Verification items for the finished model (mm, model axes). Face numbers are marked on the shaded views. A direction names the side the tool comes from. Round coordinates to 2 decimals unless told otherwise and drop trailing zeros. Loops run counter-clockwise (first coordinate to the right, second up) from the corner with the lowest first, then second, coordinate; pieces in that order, holes last. Notation, with made-up numbers: M -18.5,31.5 L -6.5,31.5 A29 ccw -6.5,67.5 Z; hole C 86,-24.5 d1. An arc over 180 degrees is marked long. Answer as CSV lines item,"result".
```python
from build123d import *

# Parameters (mm, degrees)
T_LE_DE_BASE_PLI_E1_DEPTH             = 20.5
ESQUISSE8_W                           = 24
ESQUISSE8_H                           = 2
BOSS_EXTRU_1_DEPTH                    = 8.5
T_LE_PLI_E_SUR_AR_TE1_STRIP_W         = 10
T_LE_PLI_E_SUR_AR_TE1_STRIP_H         = 2
T_LE_PLI_E_SUR_AR_TE1_STRIP_CUT_DEPTH = 8.5
T_LE_PLI_E_SUR_AR_TE1_DEPTH           = 8.5
ESQUISSE12_W                          = 1.5
ESQUISSE12_H                          = 12
ENL_V_MAT_EXTRU_1_DEPTH               = 8.5
DIAM_TRE_DU_PER_AGE_4_0_4_1_D         = 4
DIAM_TRE_DU_PER_AGE_4_0_4_2_D         = 4
CONG_1_R                              = 4
DIAM_TRE_DU_PER_AGE_8_0_8_2_D         = 8
DIAM_TRE_DU_PER_AGE_2_5_2_5_3_D       = 2.5
R_P_TITION_CIRCULAIRE2_COUNT          = 4


# Sheet-metal steps are written as plain solids
with BuildPart() as part:
    # Esquisse1 → Tôle de base pliée1 (new body)
    with BuildSketch(Plane(origin=(0, 0, 0), x_dir=(0, 0, -1), z_dir=(1, 0, 0))):
        with BuildLine():
            Line((0, 27), (0, 3))
            ThreePointArc((0, 3), (-0.878679656, 0.878679656), (-3, 0))
            Line((-3, 0), (-37.5, 0))
            Line((-37.5, 0), (-37.5, 2))
            Line((-37.5, 2), (-3, 2))
            ThreePointArc((-3, 2), (-2.292893219, 2.292893219), (-2, 3))
            Line((-2, 3), (-2, 27))
            Line((-2, 27), (0, 27))
        make_face()
    extrude(amount=T_LE_DE_BASE_PLI_E1_DEPTH)

    # Esquisse8 → Boss.-Extru.1 (add)
    with BuildSketch(Plane(origin=(20.5, 0, 0), x_dir=(0, 0, -1), z_dir=(1, 0, 0))):
        with Locations((-19, 1)):
            Rectangle(ESQUISSE8_W, ESQUISSE8_H)
    extrude(amount=BOSS_EXTRU_1_DEPTH)

    # Tôle pliée sur arête1 strip (across the edge) → Tôle pliée sur arête1 strip cut (cut)
    with BuildSketch(Plane(origin=(20.5, 2, 31), x_dir=(0, 0, -1), z_dir=(1, 0, 0))):
        with Locations((-4, -1)):
            Rectangle(T_LE_PLI_E_SUR_AR_TE1_STRIP_W, T_LE_PLI_E_SUR_AR_TE1_STRIP_H)
    extrude(amount=T_LE_PLI_E_SUR_AR_TE1_STRIP_CUT_DEPTH, mode=Mode.SUBTRACT)

    # Tôle pliée sur arête1 section (across the edge) → Tôle pliée sur arête1 (add)
    with BuildSketch(Plane(origin=(20.5, 2, 31), x_dir=(0, 0, -1), z_dir=(1, 0, 0))):
        with BuildLine():
            Line((-2, 1), (-2, 25))
            Line((-2, 25), (0, 25))
            Line((0, 25), (0, 1))
            ThreePointArc((0, 1), (0.292893219, 0.292893219), (1, 0))
            Line((1, 0), (1, -2))
            ThreePointArc((1, -2), (-1.121320344, -1.121320344), (-2, 1))
        make_face()
    extrude(amount=T_LE_PLI_E_SUR_AR_TE1_DEPTH)

    # Esquisse12 → Enlèv. mat.-Extru.1 (cut)
    with BuildSketch(Plane(origin=(0, 2, 0), x_dir=(1, 0, 0), z_dir=(0, 1, 0))):
        with Locations((19.75, -31.5)):
            Rectangle(ESQUISSE12_W, ESQUISSE12_H)
    extrude(amount=-ENL_V_MAT_EXTRU_1_DEPTH, mode=Mode.SUBTRACT)

    # Diamètre du perçage Ø4.0 (4)1 (through all)
    with Locations(Plane(origin=(0, 2, 0), x_dir=(1, 0, 0), z_dir=(0, 1, 0))):
        with Locations((24.25, -12.13), (24.25, -22.13)):
            Hole(DIAM_TRE_DU_PER_AGE_4_0_4_1_D / 2)

    # Diamètre du perçage Ø4.0 (4)2 (through all)
    with Locations(Plane.XY.offset(33)):
        with Locations((24.25, 19.87), (24.25, 9.87)):
            Hole(DIAM_TRE_DU_PER_AGE_4_0_4_2_D / 2)

    # Congé1
    cong_1_edges = [part.edges().sort_by_distance(p)[0] for p in [
        (20.5, 27, 1),
        (29, 1, 7),
        (29, 27, 32),
        (19, 1, 37.5),
    ]]
    fillet(cong_1_edges, radius=CONG_1_R)

    # Symétrie1: part across plane


with BuildPart() as part_1:
    add(part.part)
    add(part.part.mirror(Plane(origin=(0, 3, 3), x_dir=(0, 0, 1), z_dir=(1, 0, 0))))

    # Diamètre du perçage Ø8.0 (8)2 (through all)
    with Locations(Plane(origin=(0, 2, 0), x_dir=(1, 0, 0), z_dir=(0, 1, 0))):
        with Locations((0, -12.13)):
            Hole(DIAM_TRE_DU_PER_AGE_8_0_8_2_D / 2)

    # Diamètre du perçage Ø2.5 (2.5)3 (through all)
    with Locations(Plane(origin=(0, 2, 0), x_dir=(1, 0, 0), z_dir=(0, 1, 0))):
        with Locations((0, -5.13)):
            diam_tre_du_per_age_2_5_2_5_3 = Hole(DIAM_TRE_DU_PER_AGE_2_5_2_5_3_D / 2)

    # Répétition circulaire2: Diamètre du perçage Ø2.5 (2.5)3 ×4 about axis
    r_p_tition_circulaire2_axis = Axis((0, 0, 12.13), (0, 1, 0))
    for i in range(1, R_P_TITION_CIRCULAIRE2_COUNT):
        add(diam_tre_du_per_age_2_5_2_5_3.rotate(r_p_tition_circulaire2_axis, i * 360 / R_P_TITION_CIRCULAIRE2_COUNT), mode=Mode.SUBTRACT)


solid = part_1.part
```
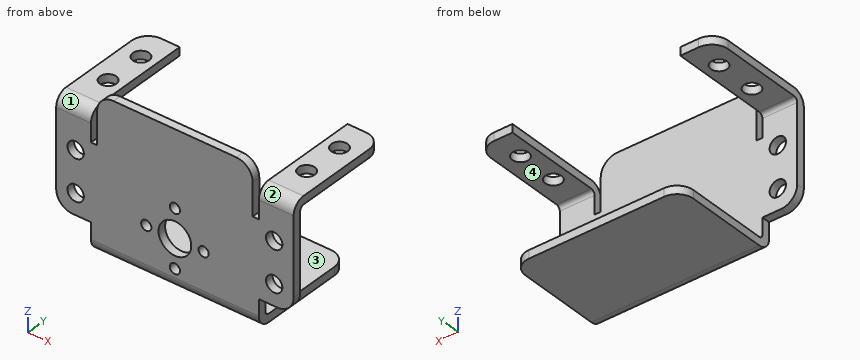
1) Section check C-C (x = -24.25). Record the cut outline in (y, z), plus the area to 3 significant figures.
Here are the results:
outline,"M 0,7 L 2,7 L 2,10.13 L 0,10.13 Z; M 0,14.13 L 2,14.13 L 2,20.13 L 0,20.13 Z; M 0,24.13 L 2,24.13 L 2,30 A1 cw 3,31 L 7.87,31 L 7.87,33 L 3,33 A3 ccw 0,30 Z; M 11.87,31 L 17.87,31 L 17.87,33 L 11.87,33 Z; M 21.87,31 L 27,31 L 27,33 L 21.87,33 Z"
area,"68.3 mm^2"
2) Material ranges on probe 1 along X at (y, z) = (1.1, 22.13); probe 2 along Y at (x, z) = (24.25, 32.4); probe 3 along Y at (x, z) = (24.25, 32.05), recorded low to high.
Here are the results:
probe 1,"x = -29 to -26.25, -22.25 to 22.25, 26.25 to 29"
probe 2,"y = 1.2 to 7.87, 11.87 to 17.87, 21.87 to 27"
probe 3,"y = 0.81 to 7.87, 11.87 to 17.87, 21.87 to 27"
3) Set-up check for the marked faces 1, 2, 3 and 4: record each of +Z, -Z, +X, -X, +Y, -Y from which the full face is reachable in a straight line by a thin tool's end or side.
Here are the results:
face 1,"+Z, -X, -Y"
face 2,"+Z, +X, -Y"
face 3,"+Z, +X, -X, +Y"
face 4,"-Z, +X, -X, +Y"
4) Section check A-A (z = 5.13). Record the cut outline in (x, y), plus the area to 3 significant figures.
Here are the results:
outline,"M -20.5,0 L -1.25,0 L -1.25,2 L -20.5,2 Z; M 1.25,0 L 20.5,0 L 20.5,2 L 1.25,2 Z"
area,"77.0 mm^2"
5) Go/stop test with flat-tipped pins: pin 1 (6.5 mm diameter, centred on x = -24.25, y = 19.87, fed in from -Z); pin 2 (2.5 mm diameter, centred on x = 26.5, y = 15, fed in from +Z); pin 3 (1 mm diameter, centred on x = -17, y = 22, fed in from +Z). Record where each tip stops, or that it passes through.
Here are the results:
pin 1,"stops at z = 31"
pin 2,"stops at z = 33"
pin 3,"stops at z = 2"
6) Section check D-D (y = 19.87). Record the cut outline in (x, z), plus the area to 3 significant figures.
Here are the results:
outline,"M -29,31 L -26.25,31 L -26.25,33 L -29,33 Z; M -22.25,31 L -20.5,31 L -20.5,33 L -22.25,33 Z; M -20.5,0 L 20.5,0 L 20.5,2 L -20.5,2 Z; M 20.5,31 L 22.25,31 L 22.25,33 L 20.5,33 Z; M 26.25,31 L 29,31 L 29,33 L 26.25,33 Z"
area,"100 mm^2"
7) Section check B-B (y = 13.5). Record the cut outline in (x, z).
Here are the results:
outline,"M -29,31 L -20.5,31 L -20.5,33 L -29,33 Z; M -20.5,0 L 20.5,0 L 20.5,2 L -20.5,2 Z; M 20.5,31 L 29,31 L 29,33 L 20.5,33 Z"
